```python
from build123d import *

# Parameters (mm, degrees)
BOSS_EXTRUDE1_DEPTH  = 1
BOSS_EXTRUDE2_DEPTH  = 2
FILLET1_R            = 1
SKETCH2_R            = 1.5
CUT_EXTRUDE1_DEPTH   = 18.790446875
M3_CLEARANCE_HOLE1_D = 3.4


with BuildPart() as part:
    # Sketch1 → Boss-Extrude1 (new body)
    with BuildSketch(Plane.XY):
        with BuildLine():
            Line((7.5, 8.5), (7.5, 12.5))
            Line((7.5, 12.5), (-12.5, 12.5))
            Line((-12.5, 12.5), (-12.5, -7.5))
            Line((-12.5, -7.5), (-8.5, -7.5))
            ThreePointArc((-8.5, -7.5), (-7.792893219, -7.792893219), (-7.5, -8.5))
            Line((-7.5, -8.5), (-7.5, -12.5))
            Line((-7.5, -12.5), (12.5, -12.5))
            Line((12.5, -12.5), (12.5, 7.5))
            Line((12.5, 7.5), (8.5, 7.5))
            ThreePointArc((8.5, 7.5), (7.792893219, 7.792893219), (7.5, 8.5))
        make_face()
        with BuildLine():
            Line((12.5, 12.5), (7.5, 12.5))
            Line((7.5, 12.5), (7.5, 8.5))
            ThreePointArc((7.5, 8.5), (7.792893219, 7.792893219), (8.5, 7.5))
            Line((8.5, 7.5), (12.5, 7.5))
            Line((12.5, 7.5), (12.5, 12.5))
        make_face()
        with BuildLine():
            Line((-8.5, -7.5), (-12.5, -7.5))
            Line((-12.5, -7.5), (-12.5, -12.5))
            Line((-12.5, -12.5), (-7.5, -12.5))
            Line((-7.5, -12.5), (-7.5, -8.5))
            ThreePointArc((-7.5, -8.5), (-7.792893219, -7.792893219), (-8.5, -7.5))
        make_face()
    extrude(amount=BOSS_EXTRUDE1_DEPTH)

    # Sketch1_3 → Boss-Extrude2 (add)
    with BuildSketch(Plane.XY):
        with BuildLine():
            Line((7.5, 8.5), (7.5, 12.5))
            Line((7.5, 12.5), (-12.5, 12.5))
            Line((-12.5, 12.5), (-12.5, -7.5))
            Line((-12.5, -7.5), (-8.5, -7.5))
            ThreePointArc((-8.5, -7.5), (-7.792893219, -7.792893219), (-7.5, -8.5))
            Line((-7.5, -8.5), (-7.5, -12.5))
            Line((-7.5, -12.5), (12.5, -12.5))
            Line((12.5, -12.5), (12.5, 7.5))
            Line((12.5, 7.5), (8.5, 7.5))
            ThreePointArc((8.5, 7.5), (7.792893219, 7.792893219), (7.5, 8.5))
        make_face()
    extrude(amount=BOSS_EXTRUDE2_DEPTH)

    # Fillet1
    fillet1_edges = [part.edges().sort_by_distance(p)[0] for p in [
        (12.5, -12.5, 1),
        (-12.5, -12.5, 0.5),
        (-12.5, 12.5, 1),
        (12.5, 12.5, 0.5),
    ]]
    fillet(fillet1_edges, radius=FILLET1_R)

    # Sketch2 → Cut-Extrude1 (cut, through all)
    with BuildSketch(Plane.XY.offset(2)):
        Circle(SKETCH2_R)
    extrude(amount=-CUT_EXTRUDE1_DEPTH, mode=Mode.SUBTRACT)

    # M3 Clearance Hole1 (through all)
    with Locations(Plane.XY.offset(1)):
        with Locations((10.5, 10.5), (-9.5, -9.5)):
            Hole(M3_CLEARANCE_HOLE1_D / 2)


solid = part.part
```
Model file for the job. Use its own axes, mm. A direction names the side the tool comes from. Coordinates: 2 decimals unless noted, no trailing zeros. Write each loop counter-clockwise with the first axis right and the second up, starting at its lowest first coordinate (ties: lowest second). Pieces come first, ordered by that corner, then holes. Notation, with made-up numbers: (16, -14.75) - (75, -14.75) arc R9 ccw to (75, -6.75) - close; hole circle Ø9 at (53, -1). An arc over 180 degrees is marked (long way). Use a Markdown table: item, result. Add a question column.
Item 1: Band-saw the part on A-A, the plane x = -9.5. Write the cut outline in (y, z).
Item 2: Drop flat-ended pins along their axis: pin 1 (0.5 mm diameter, centred on y = -9.5, z = 1.5, fed in from -X); pin 2 (0.5 mm diameter, centred on x = 10, z = 1.5, fed in from +Y); pin 3 (2.5 mm diameter, centred on x = 0, y = 0, fed in from -Z); pin 4 (2.5 mm diameter, centred on x = -10, y = -11, fed in from +Z). Give the stop position or say it passes through.
Item 3: Band-saw the part on D-D, the plane y = 10.5. Write the cut outline in (x, z), and give its area (3 significant figures).
Item 4: Band-saw the part on C-C, the plane z = 1.55. Write the cut outline in (x, y), and give its area (3 significant figures).
Item 5: Band-saw the part on B-B, the plane y = 0. Write the cut outline in (x, z), and give its area (3 significant figures).
Item 6: 3-axis set-ups, long thin cutter, end or side, ignore diameter. For faces 1 (the face through (0, -12.5, 1)), 2 (the face through (9, 9, 1)), 3 (the face through (-10.5, -7.5, 1.5)): which of +Z, -Z, +X, -X, +Y, -Y reach the whole face in a straight line?
Item 7: Two-plate mould, pull along X, no slides. Class faces 4 (the face through (-7.801, -7.785, 1.493)), 5 (the face through (0, 3, 2)), 6 (the face through (-9.13, -11.16, 0.49)): pulls with the +X half, pulls with the -X half, needs draft (parallel to the pull), parting line crosses it, or undercut.
Item 8: Drill centre lines: line 1 along Y through (x, z) = (0, 0.7); line 2 along Y through (x, z) = (-9.5, 0.4); line 3 along Y through (x, z) = (-9.5, 1.65). Where is each one in solid material? Low to high.
A:
| question | item | result |
|---|---|---|
| 1 | outline | (-12.5, 0) - (-11.2, 0) - (-11.2, 1) - (-12.5, 1) - close; (-7.8, 0) - (12.5, 0) - (12.5, 2) - (-7.5, 2) - (-7.5, 1) - (-7.8, 1) - close |
| 2 | pin 1 | stops at x = -7.5 |
| 2 | pin 2 | stops at y = 7.5 |
| 2 | pin 3 | passes through |
| 2 | pin 4 | stops at z = 1 |
| 3 | outline | (-12.5, 0) - (8.8, 0) - (8.8, 1) - (7.5, 1) - (7.5, 2) - (-12.5, 2) - close; (12.2, 0) - (12.5, 0) - (12.5, 1) - (12.2, 1) - close |
| 3 | area | 41.6 mm² |
| 4 | outline | (-12.5, -7.5) - (-8.5, -7.5) arc R1 cw to (-7.5, -8.5) - (-7.5, -12.5) - (11.5, -12.5) arc R1 ccw to (12.5, -11.5) - (12.5, 7.5) - (8.5, 7.5) arc R1 cw to (7.5, 8.5) - (7.5, 12.5) - (-11.5, 12.5) arc R1 ccw to (-12.5, 11.5) - close; hole circle Ø3 at (0, 0) |
| 4 | area | 568 mm² |
| 5 | outline | (-12.5, 0) - (-1.5, 0) - (-1.5, 2) - (-12.5, 2) - close; (1.5, 0) - (12.5, 0) - (12.5, 2) - (1.5, 2) - close |
| 5 | area | 44.0 mm² |
| 6 | face 1 | +Z, -Z, +X, -X, -Y |
| 6 | face 2 | +Z, +X, +Y |
| 6 | face 3 | +Z, -X, -Y |
| 7 | face 4 | pulls with the -X half |
| 7 | face 5 | needs draft |
| 7 | face 6 | undercut |
| 8 | line 1 | y = -12.5 to -1.5, 1.5 to 12.5 |
| 8 | line 2 | y = -12.5 to -11.2, -7.8 to 12.5 |
| 8 | line 3 | y = -7.5 to 12.5 |
